For this review, take the finished solid that the model builds, in its own axes (mm). Give positions to 0.01 mm unless a question says otherwise; leave off trailing zeros. Write each loop counter-clockwise with the first axis right and the second up, starting at its lowest first coordinate (ties: lowest second). Pieces come first, ordered by that corner, then holes.
Q1. Insertion check: P1, Ø12, axis at x = -3.5, y = 4.5, coming from the -Z side. The pin has a flat end and moves straight along its axis. Give the tip position at first contact, or say it passes through.
Q2. We need section A-A (x = 6.25). Write out the cut boundary in (y, z).
Q3. For line 1 (Y direction, x = 4.25, z = 41.5); line 2 (X direction, y = 2.75, z = 12.5); line 3 (Y direction, x = 6.5, z = 14), list the stretches that pass through material, from the lowest coordinate up.
```python
from build123d import *

# Parameters (mm, degrees)
F1_DEPTH = 25
F2_DEPTH = 25


with BuildPart() as f1:
    # F0 (on Top) → F1 (new body)
    with BuildSketch(Plane.XY):
        with BuildLine():
            Line((3.952905, 7.36742), (-11.047095, 7.36742))
            Line((-11.047095, 7.36742), (-11.047095, -12.63258))
            Line((-11.047095, -12.63258), (8.952905, -12.63258))
            Line((8.952905, -12.63258), (8.952905, 2.36742))
            ThreePointArc((8.952905, 2.36742), (7.488439, 5.902954), (3.952905, 7.36742))
        make_face()
    extrude(amount=F1_DEPTH)

    # F1_face (on face) → F2 (join)
    with BuildSketch(Plane(origin=(-1.167861, -2.753346, 25), x_dir=(1, 0, 0), z_dir=(0, 0, 1))):
        with BuildLine():
            Line((5.120766, 10.120766), (-9.879234, 10.120766))
            Line((-9.879234, 10.120766), (-9.879234, -9.879234))
            Line((-9.879234, -9.879234), (10.120766, -9.879234))
            Line((10.120766, -9.879234), (10.120766, 5.120766))
            ThreePointArc((10.120766, 5.120766), (8.6563, 8.6563), (5.120766, 10.120766))
        make_face()
    extrude(amount=F2_DEPTH)


solid = f1.part
```
Computed:
1. P1: stops at z = 0
2. outline: (-12.63, 0) - (6.81, 0) - (6.81, 50) - (-12.63, 50) - close
3. line 1: y = -12.63 to 7.36
3. line 2: x = -11.05 to 8.94
3. line 3: y = -12.63 to 6.67
